Can you work these out from the drawing? Everything is in mm from the part's minimum corner. A direction names the side the tool comes from. Round coordinates to 2 decimals unless told otherwise and drop trailing zeros. Loops run counter-clockwise (first coordinate to the right, second up) from the corner with the lowest first, then second, coordinate; pieces in that order, holes last. Notation, with made-up numbers: (-8.5, -17) -> (24.5, -17) arc R23 ccw to (24.5, -9) -> close; hole circle Ø4 at (-0.5, 62.5). An arc over 180 degrees is marked (long way). One line per item, written item: value.
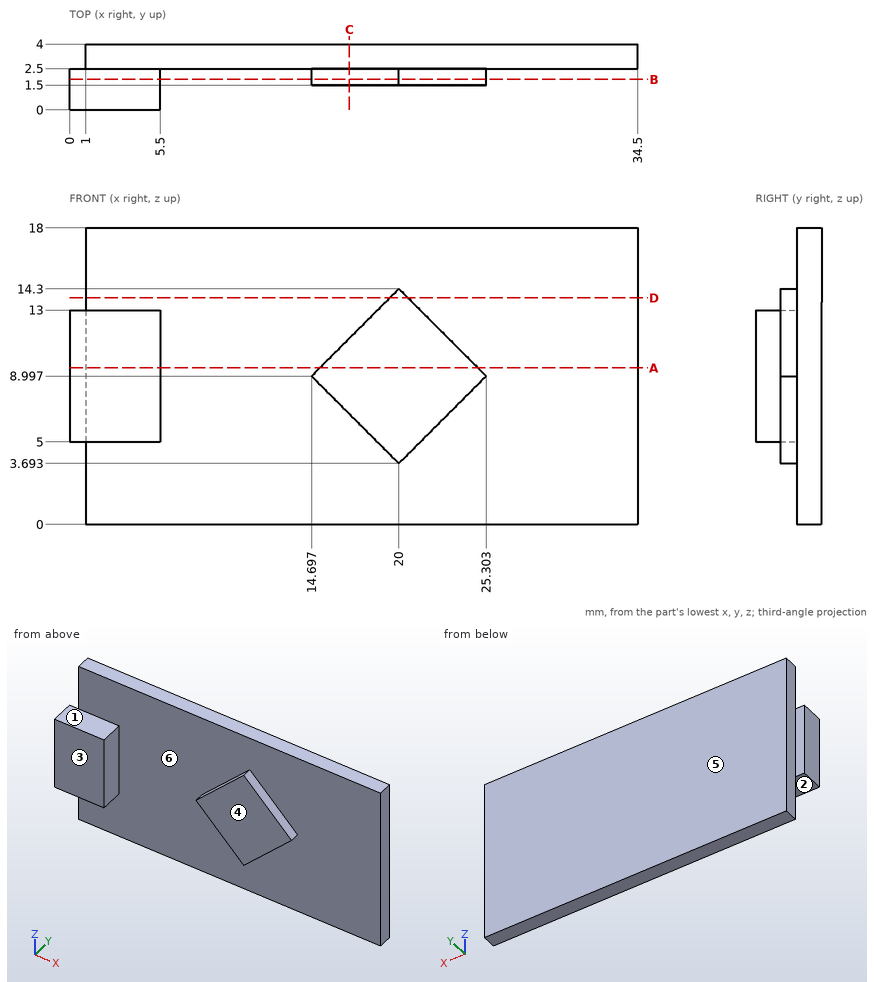
(1) For the marked faces 1, 2, 3 and 4, which set-ups out of +Z, -Z, +X, -X, +Y, -Y let a thin tool reach every point of the face, with its end or its side?
Recorded:
face 1: +Z, -X, -Y
face 2: -Z, -X, -Y
face 3: +Z, -Z, +X, -X, -Y
face 4: +Z, -Z, +X, -Y
(2) Thinking about a two-plate mould opening in X: for the marked faces 5 and 6, which applies, released by +X, released by -X, zero draft, split by the parting line, or undercut?
Recorded:
face 5: zero draft
face 6: undercut
(3) If I drill on L1, parallel to Y at x = 10, z = 4; L2, parallel to X at y = 2.55, z = 5; L3, parallel to X at y = 0.5, z = 7, over which ranges is the centre line in solid material (lowest first)?
Recorded:
L1: 2.5 to 4
L2: 1 to 34.5
L3: 0 to 5.5
(4) If we section it at B-B, the plane y = 1.85: Please give me the cut outline in (x, z), then the cut area to 3 significant figures.
Recorded:
outline: (0, 5) -> (5.5, 5) -> (5.5, 13) -> (0, 13) -> close; (14.7, 9) -> (20, 3.69) -> (25.3, 9) -> (20, 14.3) -> close
area: 100 mm²
(5) I'm going to push flat-ended pins straight in: pin 1 Ø1.3 at (y, z) = (1, 9) entering from +X; pin 2 Ø5.5 at (x, z) = (13.5, 5.5) entering from -Y; pin 3 Ø8 at (x, z) = (14, 12) entering from -Y. Where does each tip first touch, or does it pass through?
Recorded:
pin 1: x = 25.3
pin 2: y = 2.5
pin 3: y = 1.5
(6) If we section it at A-A, the plane z = 9.5: Please give me the cut outline in (x, y).
Recorded:
outline: (0, 0) -> (5.5, 0) -> (5.5, 2.5) -> (15.2, 2.5) -> (15.2, 1.5) -> (24.8, 1.5) -> (24.8, 2.5) -> (34.5, 2.5) -> (34.5, 4) -> (1, 4) -> (1, 2.5) -> (0, 2.5) -> close
(7) If we section it at C-C, the plane x = 17: Please give me the cut outline in (y, z).
Recorded:
outline: (1.5, 6.69) -> (2.5, 6.69) -> (2.5, 0) -> (4, 0) -> (4, 18) -> (2.5, 18) -> (2.5, 11.3) -> (1.5, 11.3) -> close
(8) If we section it at D-D, the plane z = 13.75: Please give me the cut outline in (x, y).
Recorded:
outline: (1, 2.5) -> (19.45, 2.5) -> (19.45, 1.5) -> (20.55, 1.5) -> (20.55, 2.5) -> (34.5, 2.5) -> (34.5, 4) -> (1, 4) -> close
